The drawing under review shows one solid part. Ordinate dimensions are in mm from its lowest x, y, z. A direction names the side the tool comes from. Round coordinates to 2 decimals unless told otherwise and drop trailing zeros. Write each loop counter-clockwise with the first axis right and the second up, starting at its lowest first coordinate (ties: lowest second). Pieces come first, ordered by that corner, then holes. Notation, with made-up numbers: (20, 13.5) - (59, 13.5) arc R21 ccw to (59, 26.5) - close; hole circle Ø4 at (-3, -23.5). An arc over 180 degrees is marked (long way). Answer in a Markdown table with one row per item. Add a question column.
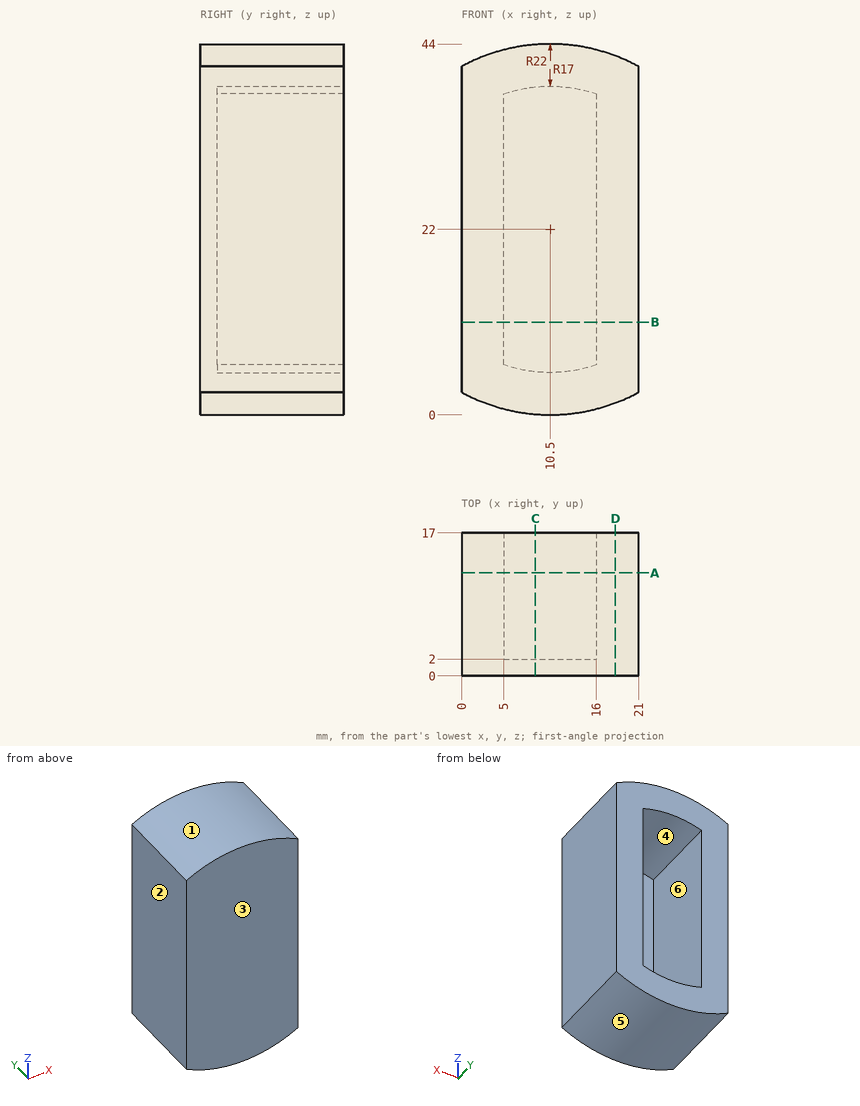
Q1. To check wall thickness, follow probe 1 along X at (y, z) = (3.5, 33.5); probe 2 along Z at (x, y) = (8, 10.25); probe 3 along Y at (x, z) = (15.5, 29.5). State the ranges of each line that lie inside material, in increasing order.
Q2. Tool access review of the marked faces 5 and 6: name each direction out of +Z, -Z, +X, -X, +Y, -Y from which nothing blocks a thin tool from reaching the whole face with its end or side.
Q3. Add section D-D on x = 18.25. State the section outline as (y, z) points, then the cut area to 3 significant figures.
Q4. Add section C-C on x = 8.75. State the section outline as (y, z) points, then the cut area to 3 significant figures.
Q5. Draft analysis for pull direction X (two halves, no side actions). For the marked faces 1, 2, 3 and 4, state which applies: released by +X, released by -X, zero draft, split by the parting line, or undercut.
Q6. Insertion check: pin 1 Ø8 at (x, z) = (4, 39) entering from -Y; pin 2 Ø5 at (x, z) = (9, 14) entering from +Y; pin 3 Ø8 at (x, y) = (4, 8) entering from +Z. Each pin has a flat end and moves straight along its axis. Give the tip position at first contact, or say it passes through.
Q7. Add section A-A on y = 12.25. State the section outline as (x, z) points, then the cut area to 3 significant figures.
Q8. Add section B-B on z = 11. State the section outline as (x, y) points, then the cut area to 3 significant figures.
Answer sheet:
| question | item | result |
|---|---|---|
| 1 | probe 1 | x = 0 to 5, 16 to 21 |
| 1 | probe 2 | z = 0.14 to 5.18, 38.82 to 43.86 |
| 1 | probe 3 | y = 0 to 2 |
| 2 | face 5 | -Z, +Y, -Y |
| 2 | face 6 | +Y |
| 3 | outline | (0, 1.41) - (17, 1.41) - (17, 42.59) - (0, 42.59) - close |
| 3 | area | 700 mm² |
| 4 | outline | (0, 0.07) - (17, 0.07) - (17, 5.09) - (2, 5.09) - (2, 38.91) - (17, 38.91) - (17, 43.93) - (0, 43.93) - close |
| 4 | area | 238 mm² |
| 5 | face 1 | split by the parting line |
| 5 | face 2 | released by -X |
| 5 | face 3 | zero draft |
| 5 | face 4 | undercut |
| 6 | pin 1 | stops at y = 0 |
| 6 | pin 2 | stops at y = 2 |
| 6 | pin 3 | stops at z = 43.86 |
| 7 | outline | (0, 2.67) arc R22 ccw to (21, 2.67) - (21, 41.33) arc R22 ccw to (0, 41.33) - close; hole (5, 5.91) arc R17 ccw to (16, 5.91) - (16, 38.09) arc R17 ccw to (5, 38.09) - close |
| 7 | area | 520 mm² |
| 8 | outline | (0, 0) - (21, 0) - (21, 17) - (16, 17) - (16, 2) - (5, 2) - (5, 17) - (0, 17) - close |
| 8 | area | 192 mm² |
